Geometry: final body of the model. Coordinates: model frame, mm. A direction names the side the tool comes from. Give positions to 0.01 mm unless a question says otherwise; leave off trailing zeros. Write each loop counter-clockwise with the first axis right and the second up, starting at its lowest first coordinate (ties: lowest second). Pieces come first, ordered by that corner, then holes. Notation, with made-up numbers: M 30.5,44.25 L 83.5,44.25 A17 ccw 83.5,77.25 Z; hole C 6,54 d4. An arc over 180 degrees is marked long. Use a Markdown table: item, result. Add a question column.
(1) Cut plane C-C (x = 3.2). State how many separate pieces and enclosed holes the cut face has, plus the area to 3 significant figures.
(2) Pin query (flat end, axial travel): pin 1 Ø1.8 at (x, z) = (3.5, -124.5) entering from +Y; pin 2 Ø1.8 at (x, z) = (4, -258.5) entering from -Y; pin 3 Ø1.5 at (x, y) = (1.5, 100.5) entering from -Z. Return the tip coordinate at first contact, or that it passes through.
(3) Reachability of faces 5 (the flat face through (0, 48, -119)), 6 (the flat face through (3, 16, -283.007)), 7 (the flat face through (3, 53, -38.1)) from +Z, -Z, +X, -X, +Y, -Y: full face, straight path, thin tool, end or side. Return the list, or none.
(4) Material intervals for L1, parallel to Z at x = 3.8, y = 21.5 (3 decimals); L2, parallel to Y at x = 3.5, z = -184.5; L3, parallel to Y at x = 0.7, z = -145.5, sorted ascending.
(5) Cut plane B-B (z = -191.5). Output: boundary loops of the cut face in (x, y).
(6) Draft query along Y for faces 1 (the cylindrical face through (3.04, 108.43, -12.29)), 2 (the flat face through (3.04, 65.23, -28.62)), 3 (the flat face through (3, 16, -25.4)), 4 (the flat face through (3.04, 34.97, -28.62)). Return one class per face: released by +Y, released by -Y, zero draft, split by the parting line, or undercut.
(7) Cut plane A-A (y = 92.58). Output: boundary loops of the cut face in (x, z) (3 decimals).
Autodesk Inventor part; units mm, degrees
ref_plane "YZ Plane" through (0, 0, 0) normal (1, 0, 0) x (0, 1, 0)
ref_plane "XZ Plane" through (0, 0, 0) normal (0, 1, 0) x (-1, 0, 0)
ref_plane "XY Plane" through (0, 0, 0) normal (0, 0, 1) x (1, 0, 0)
sketch "Sketch1" plane through (0, 0, 0) normal (1, 0, 0) x (0, 1, 0)
  line L0 (0, 0) -> (0, -38.1)
  line L1 (0, -38.1) -> (38.1, -38.1)
  line L2 (0, -308.4068) -> (0, -270.3068)
  line L3 (0, -270.3068) -> (38.1, -270.3068)
  line L4 (0, -308.4068) -> (62.1, -308.4068)
  line L5 (62.1, -308.4068) -> (62.1, -25.4)
  line L6 (62.1, -25.4) -> (138.3, -25.4)
  line L7 (138.3, -25.4) -> (138.3, 0)
  line L8 (38.1, -38.1) -> (38.1, -270.3068)
  line L9 (138.3, 0) -> (0, 0)
  line L10 (56.1, -38.1) -> (50.1, -38.1)
  line L11 (50.1, -38.1) -> (50.1, -77.1017)
  line L12 (50.1, -77.1017) -> (56.1, -77.1017)
  line L13 (56.1, -77.1017) -> (56.1, -38.1)
  line L14 (56.1, -102.5017) -> (50.1, -102.5017)
  line L15 (50.1, -102.5017) -> (50.1, -141.5034)
  line L16 (50.1, -141.5034) -> (56.1, -141.5034)
  line L17 (56.1, -141.5034) -> (56.1, -102.5017)
  line L18 (56.1, -166.9034) -> (50.1, -166.9034)
  line L19 (50.1, -166.9034) -> (50.1, -205.9051)
  line L20 (50.1, -205.9051) -> (56.1, -205.9051)
  line L21 (56.1, -205.9051) -> (56.1, -166.9034)
  line L22 (56.1, -231.3051) -> (50.1, -231.3051)
  line L23 (50.1, -231.3051) -> (50.1, -270.3068)
  line L24 (50.1, -270.3068) -> (56.1, -270.3068)
  line L25 (56.1, -270.3068) -> (56.1, -231.3051)
  point P0 (0, -289.3568)
  point P1 (56.1, -57.6008)
  point P2 (56.1, -122.0026)
  point P3 (56.1, -186.4043)
  point P4 (56.1, -250.806)
  dimension "d1" = 38.1
  dimension "d2" = 38.1
  dimension "d4" = 38.1
  dimension "d5" = 24
  dimension "d6" = 76.2
  dimension "d16" = 308.4068
  dimension "d17" = 6
  dimension "d18" = 39.0017
  dimension "d21" = 6
  dimension "d22" = 39.0017
  dimension "d23" = 25.4
  dimension "d24" = 6
  dimension "d25" = 39.0017
  dimension "d26" = 25.4
  dimension "d27" = 6
  dimension "d28" = 39.0017
  dimension "d29" = 25.4
  dimension "d49" = 25.4
  dimension "d61" = 38.1
  dimension "d62" = 50.1
extrude "Extrusion1" add sketch "Sketch1" along normal blind 6
sketch "Sketch2" plane through (0, 0, 0) normal (-1, 0, 0) x (0, 0, 1)
  circle A0 centre (-12.2165, 7.6864) radius 3.175
  circle A1 centre (-295.2013, 7.6864) radius 3.175
  point P0 (0, 0)
sketch "Sketch3" plane through (0, 0, 0) normal (-1, 0, 0) x (0, 0, 1)
  line L0 (0, 0) -> (-38.1, 0)
  line L1 (-38.1, 0) -> (-25.4, 0)
  line L2 (-25.4, 0) -> (-25.4, 38.1)
  line L3 (-25.4, 38.1) -> (-38.1, 38.1)
  line L4 (-38.1, 38.1) -> (-38.1, 0)
  line L5 (-270.3068, 38.1) -> (-270.3068, 0)
  line L6 (-270.3068, 0) -> (-283.0068, 0)
  line L7 (-283.0068, 0) -> (-283.0068, 38.1)
  line L8 (-283.0068, 38.1) -> (-270.3068, 38.1)
  line L9 (-270.3068, 38.1) -> (-270.3068, 0)
  dimension "d37" = 12.7
  dimension "d90" = 38.1
extrude "Extrusion3" cut sketch "Sketch3" against normal through all
chamfer "Chamfer1" distance 6.35 angle 45 2 edges at (3, 38.1, -283.0068) (3, 38.1, -25.4)
chamfer "Chamfer2" distance 6.35 angle 45 1 edges at (3, 62.1, -25.4)
fillet "Fillet1" radius 6.35 2 edges at (3, 138.3, -25.4) (3, 138.3, 0)
sketch "Sketch4" plane through (6, 0, 0) normal (1, 0, 0) x (0, 0, -1)
  circle A0 centre (12.7, 130.68) radius 3.175
  line L0 (19.05, 138.3) -> (6.35, 138.3)
  line L1 (25.4, 68.45) -> (25.4, 131.95)
  circle A1 centre (12.7, 117.98) radius 3.175
  circle A2 centre (12.7, 105.28) radius 3.175
  circle A3 centre (12.7, 92.58) radius 3.175
  circle A4 centre (12.7, 79.88) radius 3.175
  point P0 (0, 0)
  point P1 (12.7, 138.3)
  dimension "d50" = 6.35
  dimension "d51" = 7.62
  dimension "d54" = 12.7
sketch "Sketch5" plane through (6, 0, 0) normal (1, 0, 0) x (0, 0, -1)
  circle A0 centre (19.05, 53.1) radius 1.6256
  circle A1 centre (289.3568, 53.1) radius 1.6256
  line L0 (0, 131.95) -> (0, 0)
  line L1 (308.4068, 0) -> (308.4068, 62.1)
  line L2 (270.3068, 56.1) -> (270.3068, 50.1)
  line L3 (38.1, 50.1) -> (38.1, 56.1)
  point P0 (270.3068, 53.1)
  point P1 (38.1, 53.1)
  dimension "d63" = 3.2512
  dimension "d64" = 3.2512
  dimension "d65" = 19.05
  dimension "d66" = 19.05
hole "Hole1" at (0, 7.6864, -12.2165) at (0, 7.6864, -295.2013) direction (1, 0, 0) diameter 6.604 depth 17.0942 tip angle 118
hole "Hole2" at (6, 79.88, -12.7) at (6, 92.58, -12.7) at (6, 105.28, -12.7) at (6, 117.98, -12.7) at (6, 130.68, -12.7) direction (-1, 0, 0) diameter 6.604 depth 17.0942 tip angle 118
hole "Hole3" at (6, 53.1, -289.3568) at (6, 53.1, -19.05) direction (-1, 0, 0) diameter 4.4958 depth 17.0942 tip angle 118
sketch "Sketch6" plane through (6, 0, 0) normal (1, 0, 0) x (0, 0, -1)
  line L0 (0, 0) -> (-0.125, 0)
  line L1 (-0.125, 0) -> (-0.125, 138.3)
  line L2 (-0.125, 138.3) -> (0, 138.3)
  line L3 (0, 131.95) -> (0, 0)
  line L4 (19.05, 138.3) -> (6.35, 138.3)
  line L5 (0, 138.3) -> (6.35, 138.3)
  arc A0 (6.35, 138.3) -> (0, 131.95) centre (6.35, 131.95) ccw
  line L6 (0, 131.95) -> (0, 0)
  line L7 (308.4068, 0) -> (308.4068, 62.1)
  line L8 (308.4068, 0) -> (308.5318, 0)
  line L9 (308.5318, 0) -> (308.5318, 62.1)
  line L10 (308.5318, 62.1) -> (308.4068, 62.1)
  line L11 (308.4068, 62.1) -> (308.4068, 0)
  dimension "d91" = 0.125
  dimension "d92" = 0.125
extrude "Extrusion6" add sketch "Sketch6" against normal up to surface (6 mm away)
sketch "Sketch7" plane through (6, 0, 0) normal (1, 0, 0) x (0, 0, -1)
  line L0 (38.1, 49.915) -> (77.1017, 49.915)
  line L1 (77.1017, 49.915) -> (77.1017, 56.285)
  line L2 (77.1017, 56.285) -> (38.1, 56.285)
  line L3 (38.1, 56.285) -> (38.1, 49.915)
  line L4 (102.5017, 49.915) -> (141.5034, 49.915)
  line L5 (141.5034, 49.915) -> (141.5034, 56.285)
  line L6 (141.5034, 56.285) -> (102.5017, 56.285)
  line L7 (102.5017, 56.285) -> (102.5017, 49.915)
  line L8 (166.9034, 49.915) -> (205.9051, 49.915)
  line L9 (205.9051, 49.915) -> (205.9051, 56.285)
  line L10 (205.9051, 56.285) -> (166.9034, 56.285)
  line L11 (166.9034, 56.285) -> (166.9034, 49.915)
  line L12 (231.3051, 49.915) -> (270.3442, 49.915)
  line L13 (270.3442, 49.915) -> (270.3442, 56.285)
  line L14 (270.3442, 56.285) -> (231.3051, 56.285)
  line L15 (231.3051, 56.285) -> (231.3051, 49.915)
  point P0 (0, 0)
  dimension "d95" = 6.37
  dimension "d96" = 6.37
extrude "Extrusion7" cut sketch "Sketch7" against normal through all
fillet "Fillet2" radius 6.35 1 edges at (3, 138.3, 0.125)
sketch "Sketch8" plane through (6, 0, 0) normal (1, 0, 0) x (0, 0, -1)
  circle A0 centre (19.05, 53.1) radius 2.2479
  circle A1 centre (19.05, 53.1) radius 2.123
  circle A2 centre (289.3568, 53.1) radius 2.2479
  circle A3 centre (289.3568, 53.1) radius 2.123
  circle A4 centre (12.2165, 7.6864) radius 3.302
  circle A5 centre (12.2165, 7.6864) radius 3.177
  circle A6 centre (289.3568, 53.1) radius 8.2692
  circle A7 centre (19.05, 53.1) radius 5.3993
  circle A8 centre (12.2165, 7.6864) radius 6.0183
  circle A9 centre (295.2013, 7.6864) radius 3.302
  circle A10 centre (295.2013, 7.6864) radius 3.177
  circle A11 centre (295.2013, 7.6864) radius 6.2668
  circle A12 centre (12.7, 79.88) radius 3.302
  circle A13 centre (12.7, 79.88) radius 3.177
  circle A14 centre (12.7, 79.88) radius 5.8929
  circle A15 centre (12.7, 92.58) radius 3.302
  circle A16 centre (12.7, 92.58) radius 3.177
  circle A17 centre (12.7, 92.58) radius 5.9761
  circle A18 centre (12.7, 105.28) radius 3.302
  circle A19 centre (12.7, 105.28) radius 3.177
  circle A20 centre (12.7, 105.28) radius 5.9666
  circle A21 centre (12.7, 117.98) radius 3.302
  circle A22 centre (12.7, 117.98) radius 3.177
  circle A23 centre (12.7, 117.98) radius 6.163
  circle A24 centre (12.7, 130.68) radius 6.466
  circle A25 centre (12.7, 130.68) radius 3.177
  point P0 (0, 0)
  dimension "d100" = 4.246
  dimension "d101" = 4.246
  dimension "d102" = 6.354
  dimension "d103" = 6.354
  dimension "d104" = 6.354
  dimension "d105" = 6.354
  dimension "d106" = 6.354
  dimension "d107" = 6.354
  dimension "d108" = 6.354
extrude "Extrusion8" add sketch "Sketch8" against normal up to surface (6 mm away) contours A0 | A2 | A4 | A6 | A7 | A8 | A9 | A11 | A12 | A14 | A15 | A17 | A18 | A20 | A21 | A23 | A24
sketch "Sketch9" plane through (6, 0, 0) normal (1, 0, 0) x (0, 0, -1)
  line L0 (38.1, 55.9132) -> (77.1017, 55.9132)
  line L1 (77.1017, 55.9132) -> (77.1017, 50.3632)
  line L2 (77.1017, 50.3632) -> (38.1, 50.3632)
  line L3 (38.1, 50.3632) -> (38.1, 55.9132)
  line L4 (102.5017, 55.9132) -> (141.5034, 55.9132)
  line L5 (141.5034, 55.9132) -> (141.5034, 50.3632)
  line L6 (141.5034, 50.3632) -> (102.5017, 50.3632)
  line L7 (102.5017, 50.3632) -> (102.5017, 55.9132)
  line L8 (166.9034, 55.9132) -> (205.9051, 55.9132)
  line L9 (205.9051, 55.9132) -> (205.9051, 50.3632)
  line L10 (205.9051, 50.3632) -> (166.9034, 50.3632)
  line L11 (166.9034, 50.3632) -> (166.9034, 55.9132)
  line L12 (231.3051, 55.9132) -> (270.3442, 55.9132)
  line L13 (270.3442, 55.9132) -> (270.3442, 50.3632)
  line L14 (270.3442, 50.3632) -> (231.3051, 50.3632)
  line L15 (231.3051, 50.3632) -> (231.3051, 55.9132)
  line L16 (77.1017, 56.285) -> (77.1017, 49.915)
  line L17 (38.1, 49.915) -> (38.1, 56.285)
  line L18 (102.5017, 49.915) -> (102.5017, 56.285)
  line L19 (141.5034, 56.285) -> (141.5034, 49.915)
  line L20 (166.9034, 49.915) -> (166.9034, 56.285)
  line L21 (205.9051, 56.285) -> (205.9051, 49.915)
  line L22 (231.3051, 49.915) -> (231.3051, 56.285)
  line L23 (270.3442, 56.285) -> (270.3442, 49.915)
  circle A0 centre (12.7, 79.88) radius 3.177
  circle A1 centre (12.2165, 7.6864) radius 3.177
  circle A2 centre (12.7, 105.28) radius 3.177
  circle A3 centre (295.2013, 7.6864) radius 3.177
  circle A4 centre (12.7, 117.98) radius 3.177
  circle A5 centre (19.05, 53.1) radius 2.123
  circle A6 centre (12.7, 92.58) radius 3.177
  circle A7 centre (289.3568, 53.1) radius 2.123
  circle A8 centre (12.7, 130.68) radius 3.177
  line L24 (231.3051, 49.915) -> (231.3051, 56.285)
  line L25 (231.3051, 56.285) -> (270.3442, 56.285)
  line L26 (270.3442, 56.285) -> (270.3442, 49.915)
  line L27 (270.3442, 49.915) -> (231.3051, 49.915)
  arc A9 (6.225, 138.3) -> (-0.125, 131.95) centre (6.225, 131.95) ccw
  line L28 (-0.125, 131.95) -> (-0.125, 0)
  line L29 (-0.125, 0) -> (25.4, 0)
  line L30 (25.4, 0) -> (25.4, 31.75)
  line L31 (31.75, 38.1) -> (25.4, 31.75)
  line L32 (31.75, 38.1) -> (276.6568, 38.1)
  line L33 (283.0068, 31.75) -> (276.6568, 38.1)
  line L34 (283.0068, 31.75) -> (283.0068, 0)
  line L35 (283.0068, 0) -> (308.5318, 0)
  line L36 (308.5318, 0) -> (308.5318, 62.1)
  line L37 (308.5318, 62.1) -> (31.75, 62.1)
  line L38 (25.4, 68.45) -> (31.75, 62.1)
  line L39 (25.4, 68.45) -> (25.4, 131.95)
  arc A10 (25.4, 131.95) -> (19.05, 138.3) centre (19.05, 131.95) ccw
  line L40 (19.05, 138.3) -> (6.225, 138.3)
  line L41 (77.1017, 56.285) -> (77.1017, 49.915)
  line L42 (77.1017, 49.915) -> (38.1, 49.915)
  line L43 (38.1, 49.915) -> (38.1, 56.285)
  line L44 (38.1, 56.285) -> (77.1017, 56.285)
  line L45 (205.9051, 56.285) -> (205.9051, 49.915)
  line L46 (205.9051, 49.915) -> (166.9034, 49.915)
  line L47 (166.9034, 49.915) -> (166.9034, 56.285)
  line L48 (166.9034, 56.285) -> (205.9051, 56.285)
  line L49 (141.5034, 56.285) -> (141.5034, 49.915)
  line L50 (141.5034, 49.915) -> (102.5017, 49.915)
  line L51 (102.5017, 49.915) -> (102.5017, 56.285)
  line L52 (102.5017, 56.285) -> (141.5034, 56.285)
  point P0 (0, 0)
  dimension "d111" = 5.55
  dimension "d112" = 0
  dimension "d113" = 0
  dimension "d114" = 0
  dimension "d115" = 0
  dimension "d116" = 0
  dimension "d117" = 0
  dimension "d118" = 0
  dimension "d119" = 0
extrude "Extrusion9" add sketch "Sketch9" against normal blind 6 contours L17 L44 L16 L0 | L2 L16 L42 L17 | L18 L52 L19 L4 | L6 L19 L50 L18 | L20 L48 L21 L8 | L10 L21 L46 L20 | L22 L25 L23 L12 | L14 L23 L27 L22
equation "\"d108\" = d107"
properties part number "V3 Mounting Wall"
Answer list:
| question | item | result |
|---|---|---|
| 1 | separate pieces | 1 |
| 1 | enclosed holes | 13 |
| 1 | area | 10,200 mm² |
| 2 | pin 1 | y = 62.1 |
| 2 | pin 2 | y = 38.1 |
| 2 | pin 3 | z = -25.4 |
| 3 | face 5 | +Z, -Z, -X, +Y, -Y |
| 3 | face 6 | +X, -X, -Y |
| 3 | face 7 | +X, -X |
| 4 | L1 | -308.532 to -283.007, -25.4 to 0.125 |
| 4 | L2 | 38.1 to 50.36, 55.91 to 62.1 |
| 4 | L3 | 38.1 to 62.1 |
| 5 | outline | M 0,38.1 L 6,38.1 L 6,50.36 L 0,50.36 Z; M 0,55.91 L 6,55.91 L 6,62.1 L 0,62.1 Z |
| 6 | face 1 | undercut |
| 6 | face 2 | released by +Y |
| 6 | face 3 | zero draft |
| 6 | face 4 | released by -Y |
| 7 | outline | M 0,-25.4 L 6,-25.4 L 6,-15.877 L 0,-15.877 Z; M 0,-9.523 L 6,-9.523 L 6,0.125 L 0,0.125 Z |
